Check sheet for the drawn part. Datum: minimum x, y, z corner. Units: mm. A direction names the side the tool comes from. Coordinates: 2 decimals unless noted, no trailing zeros. Write each loop counter-clockwise with the first axis right and the second up, starting at its lowest first coordinate (ties: lowest second). Pieces come first, ordered by that corner, then holes. Notation, with made-up numbers: (-1.75, -25.75) -> (50.25, -25.75) arc R18 ccw to (50.25, -16.75) -> close; hole circle Ø8 at (4, -23). An arc over 180 degrees is marked (long way). Write each question's results on one line, items separated by ' | '. Start each with the question number.
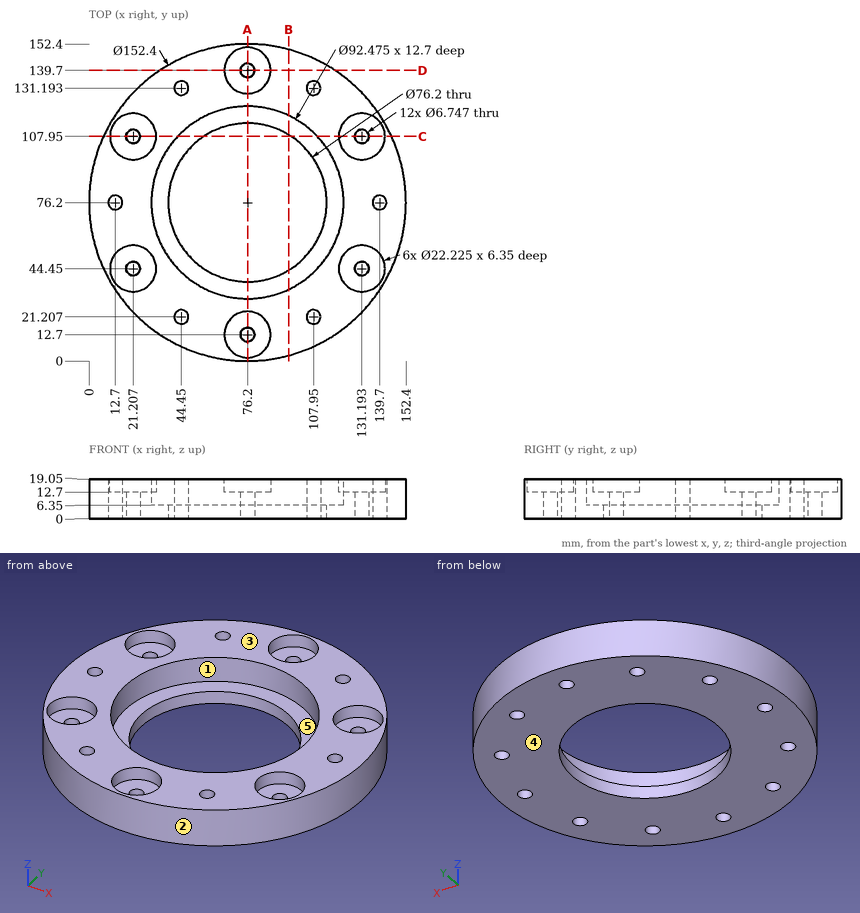
1. Sectioned sample at D-D on y = 139.7. Record the cut outline in (x, z), plus the area to 3 significant figures.
2. Material ranges on probe 1 along Y at (x, z) = (76.2, 6); probe 2 along Y at (x, z) = (77, 14) (1 decimal); probe 3 along X at (y, z) = (44.45, 6.5) (1 decimal), recorded low to high. Write a range as from..to.
3. Sectioned sample at A-A on x = 76.2. Record the cut outline in (y, z).
4. Mould release check, pull along X, two halves, no side actions. Record for the marked faces 1, 2 and 3: +X half, -X half, draft (parallel to the pull), parting line (faces both ways), or undercut.
5. Sectioned sample at C-C on y = 107.95. State how many separate pieces and enclosed holes the cut face has, plus the area to 3 significant figures.
6. Tool access check on the marked faces 4 and 5. Record the directions out of +Z, -Z, +X, -X, +Y, -Y that give a thin tool (end or side, any length) a straight path to the whole face; none if there is none.
7. Depth check by flat-ended pin: pin 1 Ø6.5 at (x, y) = (136, 47) entering from +Z; pin 2 Ø2 at (y, z) = (58.5, 9.5) entering from -X; pin 3 Ø5 at (y, z) = (29.5, 10.5) entering from +X. Enter the tip coordinate at first touch or a pass-through.
8. Sectioned sample at B-B on x = 96. Record the cut outline in (y, z), plus the area to 3 significant figures.
Computed values:
1) outline: (34.08, 0) -> (72.83, 0) -> (72.83, 12.7) -> (65.09, 12.7) -> (65.09, 19.05) -> (34.08, 19.05) -> close; (79.57, 0) -> (118.32, 0) -> (118.32, 19.05) -> (87.31, 19.05) -> (87.31, 12.7) -> (79.57, 12.7) -> close | area: 1,380 mm^2
2) probe 1: y = 0..9.33, 16.07..38.1, 114.3..136.33, 143.07..152.4 | probe 2: y = 0..1.6, 23.8..30, 122.4..128.6, 150.8..152.4 | probe 3: x = 6.9..17.8, 24.6..42.6, 109.8..127.8, 134.6..145.5
3) outline: (0, 0) -> (9.33, 0) -> (9.33, 12.7) -> (1.59, 12.7) -> (1.59, 19.05) -> (0, 19.05) -> close; (16.07, 0) -> (38.1, 0) -> (38.1, 6.35) -> (29.96, 6.35) -> (29.96, 19.05) -> (23.81, 19.05) -> (23.81, 12.7) -> (16.07, 12.7) -> close; (114.3, 0) -> (136.33, 0) -> (136.33, 12.7) -> (128.59, 12.7) -> (128.59, 19.05) -> (122.44, 19.05) -> (122.44, 6.35) -> (114.3, 6.35) -> close; (143.07, 0) -> (152.4, 0) -> (152.4, 19.05) -> (150.81, 19.05) -> (150.81, 12.7) -> (143.07, 12.7) -> close
4) face 1: undercut | face 2: parting line | face 3: draft
5) separate pieces: 4 | enclosed holes: 0 | area: 1,060 mm^2
6) face 4: -Z, +X, -X, +Y, -Y | face 5: +Z
7) pin 1: stops at z = 12.7 | pin 2: stops at x = 1.85 | pin 3: stops at x = 138.27
8) outline: (2.62, 0) -> (43.65, 0) -> (43.65, 6.35) -> (34.42, 6.35) -> (34.42, 19.05) -> (2.62, 19.05) -> close; (108.75, 0) -> (149.78, 0) -> (149.78, 19.05) -> (117.98, 19.05) -> (117.98, 6.35) -> (108.75, 6.35) -> close | area: 1,330 mm^2
